CAD build for the part. Positions are in the model's coordinates, mm. Face numbers are marked on the shaded views. Coordinates: 2 decimals unless noted, no trailing zeros. Order: outer loops, then holes, each group sorted by start corner. A loop starts at its lowest first (then second) coordinate and runs counter-clockwise, first axis right, second up. Notation, with made-up numbers: (-27, 85.25) - (-14, 85.25) arc R11 cw to (-14, 102.25) - close; hole circle Ø11 at (49, 84). An arc over 180 degrees is marked (long way). Use one line per item in the form item = value.
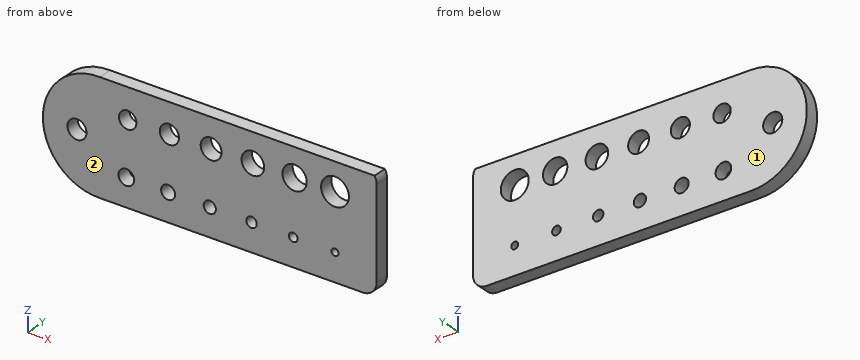
```python
from build123d import *

# Parameters (mm, degrees)
F0_R     = 4.365625
F0_R_2   = 3.571875
F0_R_3   = 3.175
F0_R_4   = 2.778125
F0_R_5   = 2.38125
F0_R_6   = 1.984375
F0_R_7   = 1.5875
F0_R_8   = 3.96875
F0_R_9   = 4.7625
F0_R_10  = 5.159375
F0_R_11  = 5.55625
F0_R_12  = 6.35
F1_DEPTH = 6.35


with BuildPart() as f1:
    # F0 (on Front) → F1 (new body)
    with BuildSketch(Plane.XZ):
        with BuildLine():
            ThreePointArc((0, 50.8), (-26.004939, 25.4), (0, 0))
            Line((0, 0), (120.045061, 0))
            ThreePointArc((120.045061, 0), (124.53519, 1.859872), (126.395061, 6.35))
            Line((126.395061, 6.35), (126.395061, 47.406904))
            ThreePointArc((126.395061, 47.406904), (126.144477, 49.173152), (125.4125, 50.8))
            Line((125.4125, 50.8), (0, 50.8))
        make_face()
        with Locations((-10.43129, 25.378589)):
            Circle(F0_R, mode=Mode.SUBTRACT)
        with Locations((12.095061, 12.7)):
            Circle(F0_R_2, mode=Mode.SUBTRACT)
        with Locations((31.145061, 12.7)):
            Circle(F0_R_3, mode=Mode.SUBTRACT)
        with Locations((50.195061, 12.7)):
            Circle(F0_R_4, mode=Mode.SUBTRACT)
        with Locations((69.245061, 12.7)):
            Circle(F0_R_5, mode=Mode.SUBTRACT)
        with Locations((88.295061, 12.7)):
            Circle(F0_R_6, mode=Mode.SUBTRACT)
        with Locations((107.345061, 12.7)):
            Circle(F0_R_7, mode=Mode.SUBTRACT)
        with Locations((12.706912, 36.952493)):
            Circle(F0_R_8, mode=Mode.SUBTRACT)
        with Locations((31.75553, 37.181994)):
            Circle(F0_R, mode=Mode.SUBTRACT)
        with Locations((50.804147, 37.411496)):
            Circle(F0_R_9, mode=Mode.SUBTRACT)
        with Locations((69.852765, 37.640997)):
            Circle(F0_R_10, mode=Mode.SUBTRACT)
        with Locations((88.901382, 37.870499)):
            Circle(F0_R_11, mode=Mode.SUBTRACT)
        with Locations((107.345061, 38.1)):
            Circle(F0_R_12, mode=Mode.SUBTRACT)
    extrude(amount=F1_DEPTH)


solid = f1.part
```
Item 1: Cut at C-C, the plane z = 5. Write the cut outline in (x, y), plus the area to 3 significant figures.
Derived:
outline = (-15.74, -6.35) - (126.25, -6.35) - (126.25, 0) - (-15.74, 0) - close
area = 902 mm²
Item 2: Drop flat-ended pins along their axis: pin 1 (10 mm diameter, centred on x = 107.35, z = 38.1, fed in from -Y) (3 decimals); pin 2 (1.5 mm diameter, centred on x = 86, y = -4, fed in from +Z); pin 3 (1.9 mm diameter, centred on x = 64, y = -4.5, fed in from -Z). Give the stop position or say it passes through.
Derived:
pin_1 = through
pin_2 = 50.8
pin_3 = 0
Item 3: Two-plate mould, pull along Y, no slides. Class the marked faces 1 and 2: +Y half, -Y half, draft (parallel to the pull), parting line (faces both ways), or undercut.
Derived:
face_1 = +Y half
face_2 = -Y half
Item 4: Cut at A-A, the plane z = 12.7. Write the cut outline in (x, y).
Derived:
outline = (-22.6, -6.35) - (8.52, -6.35) - (8.52, 0) - (-22.6, 0) - close; (15.67, -6.35) - (27.97, -6.35) - (27.97, 0) - (15.67, 0) - close; (34.32, -6.35) - (47.42, -6.35) - (47.42, 0) - (34.32, 0) - close; (52.97, -6.35) - (66.86, -6.35) - (66.86, 0) - (52.97, 0) - close; (71.63, -6.35) - (86.31, -6.35) - (86.31, 0) - (71.63, 0) - close; (90.28, -6.35) - (105.76, -6.35) - (105.76, 0) - (90.28, 0) - close; (108.93, -6.35) - (126.4, -6.35) - (126.4, 0) - (108.93, 0) - close
Item 5: Drill centre lines: line 1 (Z direction, x = 49.5, y = -2); line 2 (X direction, y = -1.5, z = 41); line 3 (Z direction, x = 23.5, y = -3). Where is each one in solid material? Low to high. Write a range as [from, to].
Derived:
line_1 = [0, 10.01], [15.39, 32.83], [41.99, 50.8]
line_2 = [-20.65, 29.64], [33.87, 47.67], [53.94, 65.94], [73.77, 84.31], [93.49, 101.7], [112.99, 126.4]
line_3 = [0, 50.8]
Item 6: Cut at B-B, the plane y = -3. State how many separate pieces and enclosed holes the cut face has, plus the area to 3 significant figures.
Derived:
separate_pieces = 1
enclosed_holes = 13
area = 6,770 mm²
